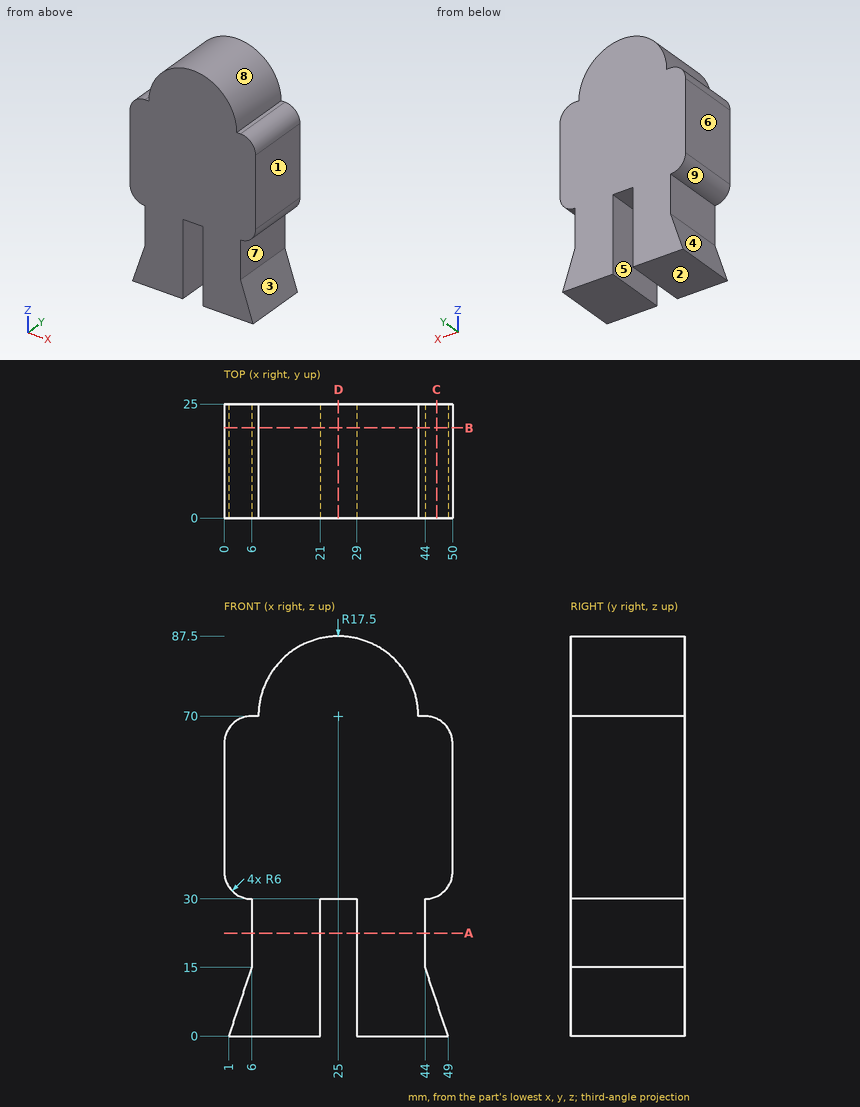
Job drawing, mm, ordinate dimensions from the low corner. One solid piece. A direction names the side the tool comes from. Give positions to 0.01 mm unless a question says otherwise; leave off trailing zeros. Loops run counter-clockwise (first coordinate to the right, second up) from the corner with the lowest first, then second, coordinate; pieces in that order, holes last. Notation, with made-up numbers: M 61,-4 L 110,-4 A17 ccw 110,20 Z; hole C -18.75,80.5 d6. An arc over 180 degrees is marked long. Use one line per item in the form item = value.
Item 1: Slice it at D-D on x = 25. List the corners of the cut face in (y, z), and give its area (3 significant figures).
Filled in:
outline = M 0,30 L 25,30 L 25,87.5 L 0,87.5 Z
area = 1,440 mm^2
Item 2: Two-plate mould, pull along Z, no slides. Class the marked faces 6, 7, 8 and 9: released by +Z, released by -Z, zero draft, split by the parting line, or undercut.
Filled in:
face_6 = zero draft
face_7 = undercut
face_8 = released by +Z
face_9 = undercut
Item 3: Which spindle directions (+Z, -Z, +X, -X, +Y, -Y) get a long thin tool onto all of the face, cutting with end or side? Do the marked faces 1, 2, 3, 4 and 5. Say none if no direction does.
Filled in:
face_1 = +Z, -Z, +X, +Y, -Y
face_2 = -Z, +X, -X, +Y, -Y
face_3 = +X, +Y, -Y
face_4 = -X, +Y, -Y
face_5 = -Z, +Y, -Y
Item 4: Drill centre lines: L1, parallel to X at y = 10.25, z = 17; L2, parallel to X at y = 9.25, z = 6; L3, parallel to Z at x = 7, y = 18.75. Where is each one in solid material? Low to high.
Filled in:
L1 = 6 to 21, 29 to 44
L2 = 3 to 21, 29 to 47
L3 = 0 to 70
Item 5: Flat gauge pins, fed straight in: pin 1 Ø5 at (y, z) = (20.5, 9) entering from +X; pin 2 Ø7.5 at (y, z) = (8, 26) entering from -X; pin 3 Ø1.2 at (x, y) = (6.5, 17) entering from +Z. Where does each tip first touch, or does it go through?
Filled in:
pin_1 = 46.83
pin_2 = 6
pin_3 = 70
Item 6: Slice it at C-C on x = 46.5. List the corners of the cut face in (y, z).
Filled in:
outline = M 0,0 L 25,0 L 25,7.5 L 0,7.5 Z; M 0,30.55 L 25,30.55 L 25,69.45 L 0,69.45 Z
Item 7: Slice it at A-A on z = 22.5. List the corners of the cut face in (x, y).
Filled in:
outline = M 6,0 L 21,0 L 21,25 L 6,25 Z; M 29,0 L 44,0 L 44,25 L 29,25 Z
Item 8: Slice it at B-B on y = 19.75. List the corners of the cut face in (x, z).
Filled in:
outline = M 0,36 A6 ccw 6,30 L 6,15 L 1,0 L 21,0 L 21,30 L 29,30 L 29,0 L 49,0 L 44,15 L 44,30 A6 ccw 50,36 L 50,64 A6 ccw 44,70 L 42.5,70 A17.5 ccw 7.5,70 L 6,70 A6 ccw 0,64 Z
